```python
from build123d import *

# Parameters (mm, degrees)
SKETCH_1_R               = 3
SKETCH_1_R_2             = 1.5
EXTRUDE_1_DEPTH          = 5
EXTRUDE_2_DEPTH          = 5
SKETCH_4_R               = 1.5
CUT_EXTRUDE_1_DEPTH      = 144.265487819
EXTRUDE_START            = -5
EXTRUDE_3_DEPTH          = 5
CUT_EXTRUDE_2_DEPTH      = 144.265487819
SKETCH_7_R               = 1.6
CUT_EXTRUDE_3_DEPTH      = 144.265487819
EXTRUDE_4_DEPTH          = 24
CUT_EXTRUDE_4_DEPTH      = 10
CUT_EXTRUDE_4_DEPTH_BACK = 144.961800489
CUT_EXTRUDE_5_DEPTH      = 144.961800489
SKETCH_14_W              = 9.91097982
SKETCH_14_H              = 20
SKETCH_14_W_2            = 10.08902018
CUT_EXTRUDE_7_DEPTH      = 146.344418537


with BuildPart() as part:
    # 草图1 → 凸台-拉伸1 (new body)
    with BuildSketch(Plane.XY):
        with BuildLine():
            Line((-3.933140204, 6.966376973), (90, 60))
            Line((90, 60), (130, 60))
            Line((130, 60), (130, 30))
            Line((130, 30), (92, 30))
            Line((92, 30), (3.100465808, -7.374761811))
            ThreePointArc((3.100465808, -7.374761811), (-7.182645896, -3.522725923), (-3.933140204, 6.966376973))
        make_face()
        Circle(SKETCH_1_R, mode=Mode.SUBTRACT)
        with Locations((95, 55)):
            Circle(SKETCH_1_R_2, mode=Mode.SUBTRACT)
        with Locations((125, 55)):
            Circle(SKETCH_1_R_2, mode=Mode.SUBTRACT)
        with Locations((125, 35)):
            Circle(SKETCH_1_R_2, mode=Mode.SUBTRACT)
        with Locations((95, 35)):
            Circle(SKETCH_1_R_2, mode=Mode.SUBTRACT)
    extrude(amount=EXTRUDE_1_DEPTH)

    # 草图3 → 凸台-拉伸2 (add)
    with BuildSketch(Plane.XY.offset(5)):
        Polygon((81.144001216, 55), (20, 55), (20, 20.478766027), align=None)
    extrude(amount=-EXTRUDE_2_DEPTH)

    # 草图4 → 切除-拉伸1 (cut, through all)
    with BuildSketch(Plane.XY.offset(5)):
        with Locations((25, 52)):
            Circle(SKETCH_4_R)
        with Locations((45, 52)):
            Circle(SKETCH_4_R)
    extrude(amount=-CUT_EXTRUDE_1_DEPTH, mode=Mode.SUBTRACT)

    # 草图6 → 凸台-拉伸3 (add)
    with BuildSketch(Plane.XY.offset(5).offset(EXTRUDE_START)):
        with BuildLine():
            Line((-7.074049095, 3.736017853), (20, 55))
            Line((20, 55), (20, 20.478766027))
            Line((20, 20.478766027), (-3.933140204, 6.966376973))
            ThreePointArc((-3.933140204, 6.966376973), (-5.735709118, 5.576884517), (-7.074049095, 3.736017853))
        make_face()
    extrude(amount=EXTRUDE_3_DEPTH)

    # 草图5 → 切除-拉伸2 (cut, through all)
    with BuildSketch(Plane.XY.offset(5)):
        with BuildLine():
            Line((25.605401824, 44.200503347), (15.042800964, 24.200503347))
            ThreePointArc((15.042800964, 24.200503347), (15.293877797, 22.454192152), (17.032531201, 22.154647985))
            Line((17.032531201, 22.154647985), (57.595132061, 42.154647985))
            ThreePointArc((57.595132061, 42.154647985), (58.392612512, 43.840567158), (56.93178603, 45))
            Line((56.93178603, 45), (26.93178603, 45))
            ThreePointArc((26.93178603, 45), (26.157433081, 44.784670195), (25.605401824, 44.200503347))
        make_face()
    extrude(amount=-CUT_EXTRUDE_2_DEPTH, mode=Mode.SUBTRACT)

    # 草图7 → 切除-拉伸3 (cut, through all)
    with BuildSketch(Plane.XY.offset(5)):
        with Locations((10, 18)):
            Circle(SKETCH_7_R)
        with Locations((30, 18)):
            Circle(SKETCH_7_R)
    extrude(amount=-CUT_EXTRUDE_3_DEPTH, mode=Mode.SUBTRACT)

    # 草图8 → 凸台-拉伸4 (add)
    with BuildSketch(Plane(origin=(130, 0, 0), x_dir=(0, 0, -1), z_dir=(1, 0, 0))):
        Polygon((0, 30), (-5, 30), (-15, 30), (-15, 60), (10, 60), (10, 30), align=None)
    extrude(amount=-EXTRUDE_4_DEPTH)

    # 草图10 → 切除-拉伸4 (cut, two sides: drawn at the far end of the back side and taken through both)
    with BuildSketch(Plane.XY.offset(5).offset(-CUT_EXTRUDE_4_DEPTH_BACK)):
        Polygon((130, 30), (130, 40), (119.91097982, 40), (92, 30), align=None)
    extrude(amount=CUT_EXTRUDE_4_DEPTH + CUT_EXTRUDE_4_DEPTH_BACK, mode=Mode.SUBTRACT)

    # 草图12 → 切除-拉伸5 (cut, through all)
    with BuildSketch(Plane.XY.offset(5)):
        with BuildLine():
            Line((40.836799147, 23.774924451), (77.710608203, 39.277253491))
            ThreePointArc((77.710608203, 39.277253491), (80.984116834, 37.94153599), (79.648399333, 34.668027359))
            Line((79.648399333, 34.668027359), (42.774590277, 19.165698319))
            ThreePointArc((42.774590277, 19.165698319), (39.501081646, 20.50141582), (40.836799147, 23.774924451))
        make_face()
    extrude(amount=-CUT_EXTRUDE_5_DEPTH, mode=Mode.SUBTRACT)

    # 草图14 → 切除-拉伸7 (cut, through all)
    with BuildSketch(Plane.XY.offset(15)):
        Polygon((106, 35.015947161), (119.91097982, 40), (110, 40), (106, 40), align=None)
        with Locations((114.95548991, 50)):
            Rectangle(SKETCH_14_W, SKETCH_14_H)
        with Locations((124.95548991, 50)):
            Rectangle(SKETCH_14_W_2, SKETCH_14_H)
    extrude(amount=-CUT_EXTRUDE_7_DEPTH, mode=Mode.SUBTRACT)


solid = part.part
```
For this review, take the finished solid that the model builds, in its own axes (mm). A direction names the side the tool comes from. Give positions to 0.01 mm unless a question says otherwise; leave off trailing zeros. Write each loop counter-clockwise with the first axis right and the second up, starting at its lowest first coordinate (ties: lowest second). Pieces come first, ordered by that corner, then holes. Notation, with made-up numbers: M -30,-8.5 L 27,-8.5 A22 cw 27,0.5 Z; hole C 45.5,-13 d5. An arc over 180 degrees is marked long. One line per item, written item: value.
1) Take a section at C-C, the plane y = 0. Write out the cut boundary in (x, z).
Results are:
outline: M -8,0 L -3,0 L -3,5 L -8,5 Z; M 3,0 L 20.64,0 L 20.64,5 L 3,5 Z
2) Take a section at B-B, the plane x = 45. Write out the cut boundary in (y, z), then the cut area to 3 significant figures.
Results are:
outline: M 10.24,0 L 20.1,0 L 20.1,5 L 10.24,5 Z; M 25.53,0 L 35.94,0 L 35.94,5 L 25.53,5 Z; M 45,0 L 50.5,0 L 50.5,5 L 45,5 Z; M 53.5,0 L 55,0 L 55,5 L 53.5,5 Z
area: 136 mm²
3) Take a section at A-A, the plane y = 52. Write out the cut boundary in (x, z), then the cut area to 3 significant figures.
Results are:
outline: M 18.42,0 L 23.5,0 L 23.5,5 L 18.42,5 Z; M 26.5,0 L 43.5,0 L 43.5,5 L 26.5,5 Z; M 46.5,0 L 106,0 L 106,-10 L 110,-10 L 110,15 L 106,15 L 106,5 L 46.5,5 Z
area: 508 mm²
4) Take a section at D-D, the plane x = 70. Write out the cut boundary in (y, z).
Results are:
outline: M 20.75,0 L 30.61,0 L 30.61,5 L 20.75,5 Z; M 36.04,0 L 55,0 L 55,5 L 36.04,5 Z
5) For faces 1 (the flat face through (106, 50, 10)), 2 (the flat face through (51, 55, 3)), 3 (the flat face through (106, 38, 3)), 4 (the flat face through (59.02, 31.42, 2.54)), list the 3-axis set-ups (+Z, -Z, +X, -X, +Y, -Y) from which the entire face can be reached by the end or side of a thin tool; tool diameter is ignored.
Results are:
face 1: +Z, -X, +Y, -Y
face 2: +Z, -Z, -X, +Y
face 3: +Z, -Z, +X, -Y
face 4: +Z, -Z
6) For P1, Ø3.5, axis at x = 30, y = 18, coming from the -Z side; P2, Ø1.5, axis at x = 41.5, z = 2.5, coming from the -Y side; P3, Ø8, axis at y = 47.5, z = 12, coming from the -X side, all flat-tipped, find the tip position at first contact; note any pin that passes through.
Results are:
P1: stops at z = 0
P2: stops at y = 8.45
P3: stops at x = 106
7) For line 1 (Y direction, x = 30.5, z = 0.25); line 2 (Y direction, x = 31, z = 2.5); line 3 (Z direction, x = 9, y = -4), list the stretches that pass through material, from the lowest coordinate up. Write a range as from..to.
Results are:
line 1: y = 4.14..16.48, 19.52..28.79, 45..55
line 2: y = 4.35..16.75, 19.25..29.04, 45..55
line 3: z = 0..5
8) The part is to be moulded in two halves that separate along X. For faces 5 (the cylindrical face through (43.8, 51.1, 2.5)), 6 (the flat face through (108, 50, -10)), 7 (the flat face through (110, 50, 3)), 8 (the flat face through (6.273, 29.009, 2.465)), say which applies: +X half, -X half, draft (parallel to the pull), parting line (faces both ways), or undercut.
Results are:
face 5: undercut
face 6: draft
face 7: +X half
face 8: -X half
